```python
from build123d import *

# Parameters (mm, degrees)
SKETCH1_R                = 15
BOSS_EXTRUDE1_DEPTH      = 35
SKETCH2_R                = 7.4
CUT_EXTRUDE1_DEPTH       = 16.6
BOSS_EXTRUDE4_REACH      = 46.179
BOSS_EXTRUDE4_END_RADIUS = 17
SKETCH5_W                = 2.5
SKETCH5_H                = 35
CIRPATTERN1_COUNT        = 34
CUT_EXTRUDE2_DEPTH       = 43.460544331
CUT_EXTRUDE2_DEPTH_BACK  = 43.460544331
SKETCH6_R                = 17
SKETCH6_R_2              = 15.5


with BuildPart() as part:
    # Sketch1 → Boss-Extrude1 (new body)
    with BuildSketch(Plane(origin=(0, 0, 0), x_dir=(1, 0, 0), z_dir=(0, 1, 0))):
        with Locations(Location((0, 0, 0), (0, 0, 270))):
            Circle(SKETCH1_R)
    extrude(amount=BOSS_EXTRUDE1_DEPTH)

    # Sketch2 → Cut-Extrude1 (cut)
    with BuildSketch(Plane(origin=(0, 35, 0), x_dir=(1, 0, 0), z_dir=(0, 1, 0))):
        with Locations(Location((0, 0, 0), (0, 0, 270))):
            Circle(SKETCH2_R)
    extrude(amount=-CUT_EXTRUDE1_DEPTH, mode=Mode.SUBTRACT)

    # Boss-Extrude4: up to this cylinder (the profile starts inside it)
    boss_extrude4_end = Plane(origin=(0, 17.5, 0), z_dir=(0, -1, 0)) * Cylinder(BOSS_EXTRUDE4_END_RADIUS, 127.358, mode=Mode.PRIVATE)
    # Sketch5 → Boss-Extrude4 (add, up to the surface)
    with BuildSketch(Plane.XY.offset(7.4), mode=Mode.PRIVATE) as boss_extrude4_sk1:
        with Locations((0, 17.5)):
            Rectangle(SKETCH5_W, SKETCH5_H)
    boss_extrude4_tool1 = extrude(boss_extrude4_sk1.sketch, amount=BOSS_EXTRUDE4_REACH, mode=Mode.PRIVATE) & boss_extrude4_end
    boss_extrude4 = boss_extrude4_tool1.solids().sort_by_distance((0, 17.5, 7.4))[0]
    add(boss_extrude4)

    # CirPattern1: Boss-Extrude4 ×34 about axis
    cirpattern1_axis = Axis((0, 0, 0), (0, 1, 0))
    for i in range(1, CIRPATTERN1_COUNT):
        add(boss_extrude4.rotate(cirpattern1_axis, i * 360 / CIRPATTERN1_COUNT))

    # Sketch6 → Cut-Extrude2 (cut, two sides: drawn at the far end of the back side and taken through both)
    with BuildSketch(Plane(origin=(0, 35, 0), x_dir=(1, 0, 0), z_dir=(0, 1, 0)).offset(-CUT_EXTRUDE2_DEPTH_BACK)):
        Circle(SKETCH6_R)
        Circle(SKETCH6_R_2, mode=Mode.SUBTRACT)
    extrude(amount=CUT_EXTRUDE2_DEPTH + CUT_EXTRUDE2_DEPTH_BACK, mode=Mode.SUBTRACT)


solid = part.part
```
Build history of the part. All positions in model axes, mm. Round coordinates to 2 decimals unless told otherwise and drop trailing zeros. Order: outer loops, then holes, each group sorted by start corner. A loop starts at its lowest first (then second) coordinate and runs counter-clockwise, first axis right, second up. Notation, with made-up numbers: (3.25, 57.25) -> (51.25, 57.25) arc R29 ccw to (51.25, 89.25) -> close; hole circle Ø8 at (75, 33). An arc over 180 degrees is marked (long way). Answer in a Markdown table with one row per item.
1) Pin check, flat tips, straight feed: P1, Ø1, axis at y = 28.5, z = 5.5, coming from the -X side; P2, Ø1, axis at y = 11.5, z = -6, coming from the +X side; P3, Ø10, axis at x = 10, y = 16, coming from the -Z side. Stop position of each tip, or through.
Values:
| item | result |
|---|---|
| P1 | x = -14.67 |
| P2 | x = 14.39 |
| P3 | z = -14.67 |
2) Mould opens along X. For faces 1 (the cylindrical face through (10.429, 17.255, 11.466)), 2 (the cylindrical face through (-7.224, 26.816, -1.604)), 3 (the cylindrical face through (-10.429, 17.255, -11.466)), 4 (the cylindrical face through (0, 17.3, -15.5)) say: released by +X, released by -X, zero draft, split by the parting line, or undercut.
Values:
| item | result |
|---|---|
| face 1 | released by +X |
| face 2 | undercut |
| face 3 | released by -X |
| face 4 | split by the parting line |
3) Band-saw the part on A-A on x = 0. Give the cut face in (y, z), and give its area (3 significant figures).
Values:
| item | result |
|---|---|
| outline | (0, -15.5) -> (35, -15.5) -> (35, -7.4) -> (18.4, -7.4) -> (18.4, 7.4) -> (35, 7.4) -> (35, 15.5) -> (0, 15.5) -> close |
| area | 839 mm2 |
4) Wall check: L1, parallel to X at y = 27.75, z = 0; L2, parallel to X at y = 24.5, z = -0.5; L3, parallel to Y at x = 3, z = 4. Give the ranges that are in metal, low to high.
Values:
| item | result |
|---|---|
| L1 | -15 to -7.4, 7.4 to 15 |
| L2 | -15.49 to -7.38, 7.38 to 15.49 |
| L3 | 0 to 18.4 |
5) Band-saw the part on B-B on x = 8. Give the cut face in (y, z), and give its area (3 significant figures).
Values:
| item | result |
|---|---|
| outline | (0, -13.28) -> (35, -13.28) -> (35, 13.28) -> (0, 13.28) -> close |
| area | 929 mm2 |
